The model under review builds one solid part; all positions refer to its coordinate system, in mm. Round coordinates to 2 decimals unless told otherwise and drop trailing zeros. Loops run counter-clockwise (first coordinate to the right, second up) from the corner with the lowest first, then second, coordinate; pieces in that order, holes last. Notation, with made-up numbers: (14, 52.25) -> (41, 52.25) arc R26 cw to (41, 75.25) -> close; hole circle Ø7 at (82, 36.25). An arc over 180 degrees is marked (long way). Return JSON: item names as keys, results as strings. Group by question number.
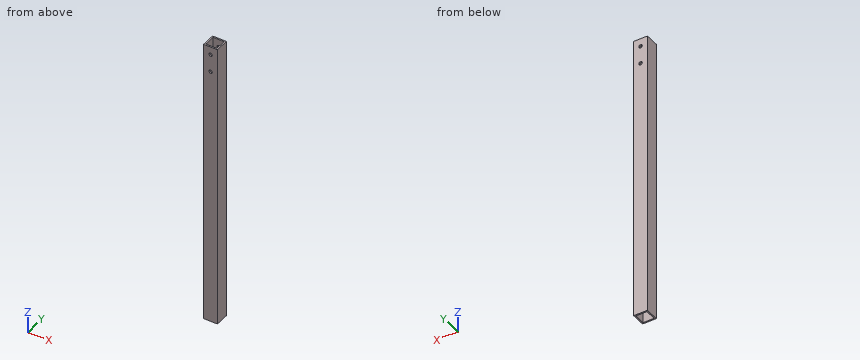
```python
from build123d import *

# Parameters (mm, degrees)
SKETCH_1_W      = 10
SKETCH_1_H      = 10
SKETCH_1_W_2    = 8
SKETCH_1_H_2    = 8
EXTRUDE_1_DEPTH = 210
HOLE_WIZARD_1_D = 2.5


with BuildPart() as part:
    # 草图1 → 凸台-拉伸1 (new body)
    with BuildSketch(Plane.XY):
        Rectangle(SKETCH_1_W, SKETCH_1_H)
        Rectangle(SKETCH_1_W_2, SKETCH_1_H_2, mode=Mode.SUBTRACT)
    extrude(amount=EXTRUDE_1_DEPTH)

    # 孔1 (through all)
    with Locations(Plane(origin=(0, -5, 0), x_dir=(-1, 0, 0), z_dir=(0, -1, 0))):
        with Locations((0, -204.177136039), (0, -191.177136039), (-130, -204.177136039), (-130, -191.177136039)):
            Hole(HOLE_WIZARD_1_D / 2)


solid = part.part
```
1. We need section A-A, the plane y = -2.25. Write out the cut boundary in (x, z).
2. We need section B-B, the plane z = 195. Write out the cut boundary in (x, y), then the cut area to 3 significant figures.
3. Wall thickness on line 1 (Z direction, x = 0, y = -4.7); line 2 (Y direction, x = -2.5, z = 100.5): over which ranges is each line inside the solid? List them lowest first.
Check sheet entries:
{
 "1": {"outline": "(-5, 0) -> (-4, 0) -> (-4, 210) -> (-5, 210) -> close; (4, 0) -> (5, 0) -> (5, 210) -> (4, 210) -> close"},
 "2": {"outline": "(-5, -5) -> (5, -5) -> (5, 5) -> (-5, 5) -> close; hole (-4, -4) -> (4, -4) -> (4, 4) -> (-4, 4) -> close", "area": "36.0 mm²"},
 "3": {"line 1": "z = 0 to 189.93, 192.43 to 202.93, 205.43 to 210", "line 2": "y = -5 to -4, 4 to 5"}
}
